Here's how the part is built. I have some questions about the finished solid (model axes, mm). Give positions to 0.01 mm unless a question says otherwise; leave off trailing zeros. Loops run counter-clockwise (first coordinate to the right, second up) from the corner with the lowest first, then second, coordinate; pieces in that order, holes last. Notation, with made-up numbers: (56.25, -26) - (91.25, -26) arc R16 ccw to (91.25, -14) - close; hole circle Ø8 at (59.25, 78.5). An arc over 180 degrees is marked (long way). Use one line per item in the form item = value.
Autodesk Fusion 360 part; units mm, degrees
sketch "Sketch1" plane through (0, 0, 0) normal (0, 0, 1) x (1, 0, 0)
  circle A0 centre (0, 0) radius 1.5
  circle A1 centre (35, 0) radius 18.5
  circle A2 centre (0, 0) radius 5
  circle A3 centre (35, 0) radius 21
  line L0 (0, -5) -> (24.6535, -18.2743)
  line L1 (0, 5) -> (24.6535, 18.2743)
  dimension "d1" = 3
  dimension "d2" = 37
  dimension "d3" = 35
  dimension "d4" = 10
  dimension "d7" = 42
  dimension "d8" = 28
  dimension "d9" = 28
extrude "Extrude1" add sketch "Sketch1" along normal blind 3
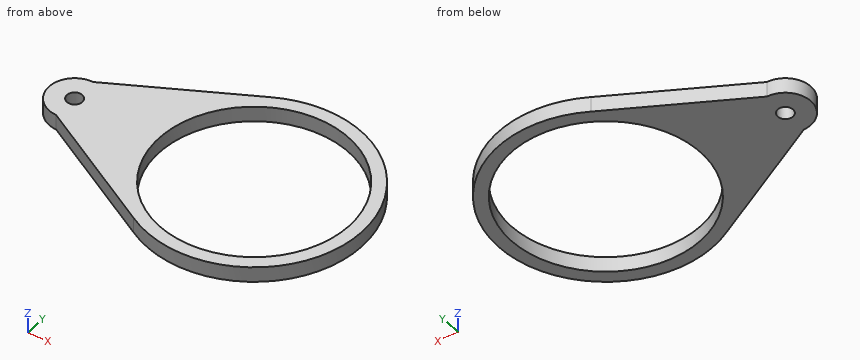
(1) If I drill on probe 1 along Y at (x, z) = (0, 1.5); probe 2 along Y at (x, z) = (35.5, 0.6); probe 3 along X at (y, z) = (8.5, 1.95), over which ranges is the centre line in solid material (lowest first)?
Geometry says:
probe_1 = -5 to -1.5, 1.5 to 5
probe_2 = -20.99 to -18.49, 18.49 to 20.99
probe_3 = 6.5 to 18.57, 51.43 to 54.2
(2) If we section it at A-A (x = 35): List the corners of the cut face in (y, z) for me.
Geometry says:
outline = (-21, 0) - (-18.5, 0) - (-18.5, 3) - (-21, 3) - close; (18.5, 0) - (21, 0) - (21, 3) - (18.5, 3) - close
(3) If we section it at C-C (z = 0.8): List the corners of the cut face in (x, y) for me.
Geometry says:
outline = (0, -5) - (24.65, -18.27) arc R21 ccw (long way) to (24.65, 18.27) - (0, 5) arc R5 ccw to start; hole circle Ø3 at (0, 0); hole circle Ø37 at (35, 0)
(4) For P1, Ø10, axis at x = 15.5, y = 13, coming from the -Z side; P2, Ø1, axis at y = 14.5, z = 1, coming from the +X side, each with a flat end and sliding along its axis, tell me the tip position at first contact or that it passes through.
Geometry says:
P1 = 0
P2 = 50.65
(5) If we section it at B-B (y = 3): List the corners of the cut face in (x, z) for me, plus the area to 3 significant figures.
Geometry says:
outline = (-4, 0) - (16.74, 0) - (16.74, 3) - (-4, 3) - close; (53.26, 0) - (55.78, 0) - (55.78, 3) - (53.26, 3) - close
area = 69.8 mm²
